from build123d import *

# Parameters (mm, degrees)
SALIENTE_EXTRUIR5_DEPTH  = 40
CORTAR_EXTRUIR3_DEPTH    = 38
CROQUIS19_R              = 16
CORTAR_EXTRUIR4_DEPTH    = 16
CROQUIS22_R              = 6
CORTAR_EXTRUIR6_DEPTH    = 16
CROQUIS25_W              = 6
CROQUIS25_H              = 16
CORTAR_EXTRUIR10_DEPTH   = 0.6
CROQUIS28_R              = 18
CORTAR_EXTRUIR11_DEPTH   = 1
SALIENTE_EXTRUIR7_DEPTH  = 4
CROQUIS30_R              = 16
CORTAR_EXTRUIR12_DEPTH   = 34
CORTAR_EXTRUIR13_START   = 3.5
CROQUIS31_R              = 18
CORTAR_EXTRUIR13_DEPTH   = 3.5
CROQUIS24_W              = 16
CROQUIS24_H              = 3
CORTAR_EXTRUIR14_DEPTH   = 1.2
CROQUIS23_W              = 16
CROQUIS23_H              = 3
CORTAR_EXTRUIR15_DEPTH   = 1.2
CROQUIS32_R              = 2.5
SALIENTE_EXTRUIR8_DEPTH  = 7
CROQUIS49_R              = 1
SALIENTE_EXTRUIR9_DEPTH  = 4.5
CROQUIS47_R              = 1
SALIENTE_EXTRUIR10_DEPTH = 4.5
CROQUIS48_R              = 1
SALIENTE_EXTRUIR11_DEPTH = 4.5
CROQUIS50_R              = 1
SALIENTE_EXTRUIR12_DEPTH = 4.5


with BuildPart() as part:
    # Croquis1 → Saliente-Extruir5 (new body)
    with BuildSketch(Plane(origin=(0, 0, 0), x_dir=(1, 0, 0), z_dir=(0, 1, 0))):
        with BuildLine():
            Line((-76.52774776, -47.188914739), (-76.52774776, 21.977990865))
            ThreePointArc((-76.52774776, 21.977990865), (-51.168030611, 47.337708015), (-25.808313462, 21.977990865))
            Line((-25.808313462, 21.977990865), (-25.808313462, -47.033075243))
            ThreePointArc((-25.808313462, -47.033075243), (-51.106035712, -67.287819919), (-76.52774776, -47.188914739))
        make_face()
    extrude(amount=SALIENTE_EXTRUIR5_DEPTH)

    # Croquis16 → Cortar-Extruir3 (cut)
    with BuildSketch(Plane(origin=(0, 40, 0), x_dir=(1, 0, 0), z_dir=(0, 1, 0))):
        with BuildLine():
            Line((-74.52774776, 21.977990865), (-74.52774776, -46.95348914))
            ThreePointArc((-74.52774776, -46.95348914), (-51.109128236, -65.287819786), (-27.808313462, -46.804003852))
            Line((-27.808313462, -46.804003852), (-27.808313462, 21.977990865))
            ThreePointArc((-27.808313462, 21.977990865), (-51.168030611, 45.337708015), (-74.52774776, 21.977990865))
        make_face()
    extrude(amount=-CORTAR_EXTRUIR3_DEPTH, mode=Mode.SUBTRACT)

    # Croquis19 → Cortar-Extruir4 (cut)
    with BuildSketch(Plane(origin=(0, 2, 0), x_dir=(1, 0, 0), z_dir=(0, 1, 0))):
        with Locations(Location((-51.168030611, 21.977990865, 0), (0, 0, 270))):
            Circle(CROQUIS19_R)
    extrude(amount=-CORTAR_EXTRUIR4_DEPTH, mode=Mode.SUBTRACT)

    # Croquis22 → Cortar-Extruir6 (cut)
    with BuildSketch(Plane(origin=(0, 2, 0), x_dir=(1, 0, 0), z_dir=(0, 1, 0))):
        with Locations(Location((-51.168030611, -14.810665764, 0), (0, 0, 270))):
            Circle(CROQUIS22_R)
    extrude(amount=-CORTAR_EXTRUIR6_DEPTH, mode=Mode.SUBTRACT)

    # Croquis25 → Cortar-Extruir10 (cut)
    with BuildSketch(Plane(origin=(0, 2, 0), x_dir=(1, 0, 0), z_dir=(0, 1, 0))):
        with Locations((-51.168030611, -14.810665764)):
            Rectangle(CROQUIS25_W, CROQUIS25_H)
    extrude(amount=-CORTAR_EXTRUIR10_DEPTH, mode=Mode.SUBTRACT)

    # Croquis28 → Cortar-Extruir11 (cut)
    with BuildSketch(Plane(origin=(0, 2, 0), x_dir=(1, 0, 0), z_dir=(0, 1, 0))):
        with Locations(Location((-51.168030611, 21.977990865, 0), (0, 0, 270))):
            Circle(CROQUIS28_R)
    extrude(amount=-CORTAR_EXTRUIR11_DEPTH, mode=Mode.SUBTRACT)

    # Croquis29 → Saliente-Extruir7 (add)
    with BuildSketch(Plane(origin=(0, 2, 0), x_dir=(1, 0, 0), z_dir=(0, 1, 0))):
        with BuildLine():
            Line((-71.168030611, 21.977990865), (-31.168030611, 21.977990865))
            ThreePointArc((-31.168030611, 21.977990865), (-51.168030611, 41.977990865), (-71.168030611, 21.977990865))
        make_face()
    extrude(amount=SALIENTE_EXTRUIR7_DEPTH)

    # Croquis30 → Cortar-Extruir12 (cut)
    with BuildSketch(Plane(origin=(0, 6, 0), x_dir=(1, 0, 0), z_dir=(0, 1, 0))):
        with Locations(Location((-51.168030611, 21.977990865, 0), (0, 0, 270))):
            Circle(CROQUIS30_R)
    extrude(amount=-CORTAR_EXTRUIR12_DEPTH, mode=Mode.SUBTRACT)

    # Croquis31 → Cortar-Extruir13 (cut)
    with BuildSketch(Plane(origin=(0, 1, 0), x_dir=(1, 0, 0), z_dir=(0, 1, 0)).offset(CORTAR_EXTRUIR13_START)):
        with Locations(Location((-51.168030611, 21.977990865, 0), (0, 0, 270))):
            Circle(CROQUIS31_R)
    extrude(amount=-CORTAR_EXTRUIR13_DEPTH, mode=Mode.SUBTRACT)

    # Croquis24 → Cortar-Extruir14 (cut)
    with BuildSketch(Plane.ZY.offset(27.808313462)):
        with Locations((-13.977990865, 35.2)):
            Rectangle(CROQUIS24_W, CROQUIS24_H)
        with Locations((38.804003852, 35.2)):
            Rectangle(CROQUIS24_W, CROQUIS24_H)
    extrude(amount=-CORTAR_EXTRUIR14_DEPTH, mode=Mode.SUBTRACT)

    # Croquis23 → Cortar-Extruir15 (cut)
    with BuildSketch(Plane(origin=(-74.52774776, 0, 0), x_dir=(0, 0, -1), z_dir=(1, 0, 0))):
        with Locations((-38.95348914, 35.2)):
            Rectangle(CROQUIS23_W, CROQUIS23_H)
        with Locations((13.977990865, 35.2)):
            Rectangle(CROQUIS23_W, CROQUIS23_H)
    extrude(amount=-CORTAR_EXTRUIR15_DEPTH, mode=Mode.SUBTRACT)

    # Croquis32 → Saliente-Extruir8 (add)
    with BuildSketch(Plane(origin=(0, 2, 0), x_dir=(1, 0, 0), z_dir=(0, 1, 0))):
        with Locations(Location((-68.12774776, -49.95348914, 0), (0, 0, 270))):
            Circle(CROQUIS32_R)
        with Locations(Location((-34.208313462, -49.804003852, 0), (0, 0, 270))):
            Circle(CROQUIS32_R)
        with Locations(Location((-68.12774776, -6.95348914, 0), (0, 0, 270))):
            Circle(CROQUIS32_R)
        with Locations(Location((-34.208313462, -6.804003852, 0), (0, 0, 270))):
            Circle(CROQUIS32_R)
    extrude(amount=SALIENTE_EXTRUIR8_DEPTH)

    # Croquis49 → Saliente-Extruir9 (add)
    with BuildSketch(Plane(origin=(0, 9, 0), x_dir=(1, 0, 0), z_dir=(0, 1, 0))):
        with Locations(Location((-34.208313462, -49.804003852, 0), (0, 0, 270))):
            Circle(CROQUIS49_R)
    extrude(amount=SALIENTE_EXTRUIR9_DEPTH)

    # Croquis47 → Saliente-Extruir10 (add)
    with BuildSketch(Plane(origin=(0, 9, 0), x_dir=(1, 0, 0), z_dir=(0, 1, 0))):
        with Locations(Location((-34.208313462, -6.804003852, 0), (0, 0, 270))):
            Circle(CROQUIS47_R)
    extrude(amount=SALIENTE_EXTRUIR10_DEPTH)

    # Croquis48 → Saliente-Extruir11 (add)
    with BuildSketch(Plane(origin=(0, 9, 0), x_dir=(1, 0, 0), z_dir=(0, 1, 0))):
        with Locations(Location((-68.12774776, -6.95348914, 0), (0, 0, 270))):
            Circle(CROQUIS48_R)
    extrude(amount=SALIENTE_EXTRUIR11_DEPTH)

    # Croquis50 → Saliente-Extruir12 (add)
    with BuildSketch(Plane(origin=(0, 9, 0), x_dir=(1, 0, 0), z_dir=(0, 1, 0))):
        with Locations(Location((-68.12774776, -49.95348914, 0), (0, 0, 270))):
            Circle(CROQUIS50_R)
    extrude(amount=SALIENTE_EXTRUIR12_DEPTH)


solid = part.part
Geometry check sheet. Reference: the model listing, model coordinates, mm. A direction names the side the tool comes from. Give positions to 0.01 mm unless a question says otherwise; leave off trailing zeros. Loops run counter-clockwise (first coordinate to the right, second up) from the corner with the lowest first, then second, coordinate; pieces in that order, holes last. Notation, with made-up numbers: (80.5, 17.25) -> (119.5, 17.25) arc R27 ccw to (119.5, 52.25) -> close; hole circle Ø8 at (0.25, 54.25). An arc over 180 degrees is marked (long way). Answer in a Markdown table with one row per item. Add a question column.
1) Cross-section at A-A on y = 35. Record the boundary of the cut face in (x, z).
2) Cross-section at D-D on y = 25. Record the boundary of the cut face in (x, z), and give its area (3 significant figures).
3) Gauge pin test, flat ends, axial feed: P1, Ø1, axis at x = -34.5, z = 6.5, coming from the +Y side; P2, Ø1.5, axis at x = -52.5, z = 7, coming from the +Y side; P3, Ø12, axis at x = -67, z = 41, coming from the -Y side; P4, Ø5, axis at x = -58.5, y = 6.5, coming from the -Z side. Record the tip position at first contact, or that the pin passes through.
4) Draft check along X on faces 4 (the face through (-50.62, 19.72, 67.28)), 5 (the face through (-27, 40, 5)), 6 (the face through (-27.808, 21, 13)). Enter one of: pulls with the +X half, pulls with the -X half, needs draft (parallel to the pull), parting line crosses it, or undercut.
5) Set-up check for faces 1 (the face through (-35.304, 0.507, -24.061)), 2 (the face through (-70, 4, -21.978)), 3 (the face through (-50.38, 2.39, -39.96)): record each of +Z, -Z, +X, -X, +Y, -Y from which the full face is reachable in a straight line by a thin tool's end or side.
6) Cross-section at B-B on z = -13. Record the boundary of the cut face in (x, y), and give its area (3 significant figures).
7) Material ranges on probe 1 along X at (y, z) = (19.5, 15); probe 2 along X at (y, z) = (36.5, 31.5); probe 3 along Z at (x, y) = (-51.5, 10), recorded low to high. Write a range as from..to.
8) Cross-section at C-C on x = -62.5. Record the boundary of the cut face in (y, z) (3 decimals).
Outcome:
| question | item | result |
|---|---|---|
| 1 | outline | (-76.53, -21.98) arc R25.36 ccw to (-25.81, -21.98) -> (-25.81, 47.03) arc R26.03 ccw to (-76.53, 47.19) -> close; hole (-75.73, -21.98) -> (-74.53, -21.98) arc R23.36 ccw to (-27.81, -21.98) -> (-26.61, -21.98) -> (-26.61, -5.98) -> (-27.81, -5.98) -> (-27.81, 30.8) -> (-26.61, 30.8) -> (-26.61, 46.8) -> (-27.81, 46.8) arc R24.03 ccw to (-74.53, 46.95) -> (-75.73, 46.95) -> (-75.73, 30.95) -> (-74.53, 30.95) -> (-74.53, -5.98) -> (-75.73, -5.98) -> close |
| 2 | outline | (-76.53, -21.98) arc R25.36 ccw to (-25.81, -21.98) -> (-25.81, 47.03) arc R26.03 ccw to (-76.53, 47.19) -> close; hole (-74.53, -21.98) arc R23.36 ccw to (-27.81, -21.98) -> (-27.81, 46.8) arc R24.03 ccw to (-74.53, 46.95) -> close |
| 2 | area | 563 mm^2 |
| 3 | P1 | stops at y = 13.5 |
| 3 | P2 | stops at y = 2 |
| 3 | P3 | stops at y = 0 |
| 3 | P4 | stops at z = -46.87 |
| 4 | face 4 | parting line crosses it |
| 4 | face 5 | needs draft |
| 4 | face 6 | undercut |
| 5 | face 1 | +Y, -Y |
| 5 | face 2 | +Y |
| 5 | face 3 | none |
| 6 | outline | (-76.53, 0) -> (-64.41, 0) -> (-64.41, 1) -> (-66.77, 1) -> (-66.77, 2) -> (-74.53, 2) -> (-74.53, 33.7) -> (-75.73, 33.7) -> (-75.73, 36.7) -> (-74.53, 36.7) -> (-74.53, 40) -> (-76.53, 40) -> close; (-37.92, 0) -> (-25.81, 0) -> (-25.81, 40) -> (-27.81, 40) -> (-27.81, 36.7) -> (-26.61, 36.7) -> (-26.61, 33.7) -> (-27.81, 33.7) -> (-27.81, 2) -> (-35.57, 2) -> (-35.57, 1) -> (-37.92, 1) -> close |
| 6 | area | 189 mm^2 |
| 7 | probe 1 | x = -76.53..-74.53, -27.81..-25.81 |
| 7 | probe 2 | x = -76.53..-75.73, -26.61..-25.81 |
| 7 | probe 3 | z = -47.34..-45.34, 65.29..67.29 |
| 8 | outline | (0, -44.665) -> (40, -44.665) -> (40, -42.405) -> (2, -42.405) -> (2, -38.458) -> (6, -38.458) -> (6, -33.273) -> (4.5, -33.273) -> (4.5, -35.963) -> (1, -35.963) -> (1, -33.273) -> (0, -33.273) -> close; (0, -10.683) -> (1, -10.683) -> (1, -7.993) -> (2, -7.993) -> (2, 62.457) -> (40, 62.457) -> (40, 64.7) -> (0, 64.7) -> close |
